Check sheet for the modelled part. Datum: model origin and axes. Units: mm. Face numbers are marked on the shaded views. A direction names the side the tool comes from. Coordinates: 2 decimals unless noted, no trailing zeros. Write each loop counter-clockwise with the first axis right and the second up, starting at its lowest first coordinate (ties: lowest second). Pieces come first, ordered by that corner, then holes. Notation, with made-up numbers: M 9.5,69.25 L 63.5,69.25 A31 ccw 63.5,97.25 Z; hole C 65.25,-29.75 d2. An arc over 180 degrees is marked long. Answer as CSV lines item,"result". Start each with the question number.
1) Access from +Z, -Z, +X, -X, +Y, -Y to the whole of each face (thin tool, end or side, straight path). Record for the marked faces 4 and 5.
2) Material ranges on L1, parallel to Y at x = 0, z = 2.1; L2, parallel to Y at x = 0, z = 1.35; L3, parallel to Z at x = -2.4, y = -1.2, recorded low to high. Write a range as [from, to].
3) Section check A-A (y = 0). Record the cut outline in (x, z), and give its area (3 significant figures).
4) Section check D-D (y = -2.45). Record the cut outline in (x, z), and give its area (3 significant figures).
5) Draft check along Y on the marked faces 1, 2 and 3. Enter one of: +Y half, -Y half, draft (parallel to the pull), parting line (faces both ways), or undercut.
6) Section check C-C (z = 2.7). Record the cut outline in (x, y).
from build123d import *

# Parameters (mm, degrees)
F0_R     = 3
F0_R_2   = 0.5
F1_DEPTH = 1.4
F2_R     = 2.2
F2_R_2   = 0.5
F3_DEPTH = 4
F4_SIZE2 = 3
F4_SIZE  = 0.2


with BuildPart() as f1:
    # F0 (on Top) → F1 (new body)
    with BuildSketch(Plane.XY):
        Circle(F0_R)
        Circle(F0_R_2, mode=Mode.SUBTRACT)
    extrude(amount=F1_DEPTH)

    # F2 (on face) → F3 (join)
    with BuildSketch(Plane.XY.offset(1.4)):
        Circle(F2_R)
        Circle(F2_R_2, mode=Mode.SUBTRACT)
    extrude(amount=F3_DEPTH)

    # F4
    f4_edges = [f1.edges().sort_by_distance(p)[0] for p in [
        (-2.2, 0, 5.4),
    ]]
    f4_side = f1.faces().sort_by_distance((-2.137775, 0, 5.4))[0]
    chamfer(f4_edges, length=F4_SIZE, length2=F4_SIZE2, reference=f4_side)


solid = f1.part
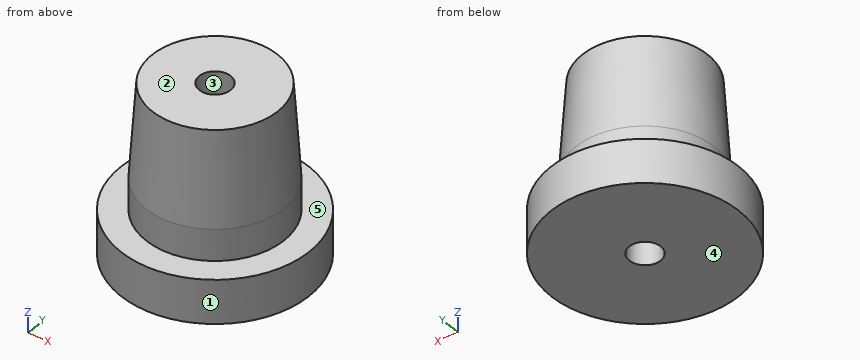
Results found:
1,face 4,"-Z, +X, -X, +Y, -Y"
1,face 5,"+Z"
2,L1,"y = [-2.2, -0.5], [0.5, 2.2]"
2,L2,"y = [-3, -0.5], [0.5, 3]"
2,L3,"z = [0, 1.4]"
3,outline,"M -3,0 L -0.5,0 L -0.5,5.4 L -2,5.4 L -2.2,2.4 L -2.2,1.4 L -3,1.4 Z; M 0.5,0 L 3,0 L 3,1.4 L 2.2,1.4 L 2.2,2.4 L 2,5.4 L 0.5,5.4 Z"
3,area,"20.0 mm2"
4,outline,"M -1.73,0 L 1.73,0 L 1.73,1.4 L -1.73,1.4 Z"
4,area,"4.85 mm2"
5,face 1,"parting line"
5,face 2,"draft"
5,face 3,"undercut"
6,outline,"C 0,0 d4.36; hole C 0,0 d1"
